Can you work these out from the model? Positions are in its coordinate system, mm. A direction names the side the tool comes from. Coordinates: 2 decimals unless noted, no trailing zeros. Write each loop counter-clockwise with the first axis right and the second up, starting at its lowest first coordinate (ties: lowest second). Pieces come first, ordered by that corner, then holes. Notation, with made-up numbers: (-7.75, 79) - (51.25, 79) arc R26 ccw to (51.25, 95) - close; hole circle Ø7 at (-1, 31). An arc over 180 degrees is marked (long way). Use one line per item in the form item = value. Start each with the question number.
(1) If I drill on probe 1 along Y at (x, z) = (0, 2); probe 2 along X at (y, z) = (-8.5, -2.5); probe 3 along X at (y, z) = (-17, 2), over which ranges is the centre line in solid material (lowest first)? Write a range as from..to.
(2) If we section it at A-A on y = -11: Please give me the cut outline in (x, z), then the cut area to 3 significant figures.
(3) If we section it at B-B on z = -2: Give the number of separate pieces and of enclosed holes in the cut face, then the cut area to 3 significant figures.
(4) Thinking about a two-plate mould opening in X: for faces 1 (the face through (14.449, 24.567, 3.586)), 2 (the face through (-3.938, -29.365, -1.972)), 3 (the face through (12.93, 21.98, 3.59)), which applies, pulls with the +X half, pulls with the -X half, needs draft (parallel to the pull), parting line crosses it, or undercut?
(5) On a 3-axis mill with a long thin cutter (end or side, diameter ignored), from which of +Z, -Z, +X, -X, +Y, -Y can I reach the whole of each face in a straight line? I mean faces 4 (the face through (12.572, -22.187, 3.586)), 5 (the face through (17.749, 20.954, 2.098)), 6 (the face through (27, 0, 3)), 7 (the face through (-27.4, -11, -2)), 8 (the face through (3.583, 28.415, -1.972)). Say none if no direction works.
(6) If we section it at D-D on y = -3.5: Please give me the cut outline in (x, z), then the cut area to 3 significant figures.
(7) If we section it at C-C on x = -3.5: Please give me the cut outline in (y, z).
(8) For pin 1 Ø0.9 at (x, y) = (27, 1) entering from -Z; pin 2 Ø2 at (y, z) = (9, -2) entering from +X; pin 3 Ø1.2 at (y, z) = (-10, -2.5) entering from -X, each with a flat end and sliding along its axis, tell me the tip position at first contact or that it passes through.
```python
from build123d import *

# Parameters (mm, degrees)
BOSS_EXTRUDE1_DEPTH = 4.34
CUT_EXTRUDE1_DEPTH  = 66.960864154
CUT_EXTRUDE2_REACH  = 73.855
CUT_EXTRUDE3_REACH  = 73.855
BOSS_EXTRUDE2_DEPTH = 4


with BuildPart() as part:
    # Sketch1 → Boss-Extrude1 (new body)
    with BuildSketch(Plane(origin=(0, 0, 0), x_dir=(0, 1, 0), z_dir=(0, 0, 1))):
        Polygon((32.908965344, 0), (16.454482672, 28.5), (-16.454482672, 28.5), (-32.908965344, 0), (-16.454482672, -28.5), (16.454482672, -28.5), align=None)
        Polygon((29.444863729, 0), (14.722431864, 25.5), (-14.722431864, 25.5), (-29.444863729, 0), (-14.722431864, -25.5), (14.722431864, -25.5), align=None, mode=Mode.SUBTRACT)
    extrude(amount=BOSS_EXTRUDE1_DEPTH)

    # Sketch2 → Cut-Extrude1 (cut, through all)
    with BuildSketch(Plane.YZ.offset(28.5)):
        with BuildLine():
            Line((-2.75, 3), (2.75, 3))
            ThreePointArc((2.75, 3), (5.75, 0), (2.75, -3))
            Line((2.75, -3), (-2.75, -3))
            ThreePointArc((-2.75, -3), (-5.75, 0), (-2.75, 3))
        make_face()
    extrude(amount=-CUT_EXTRUDE1_DEPTH, mode=Mode.SUBTRACT)

    # Cut-Extrude2: up to this face of the body (flat: up to its plane)
    cut_extrude2_end = Plane(part.part.faces().sort_by_distance((-14.25, -24.681724008, 2.17))[0])
    # Sketch3 → Cut-Extrude2 (cut, up to the picked face)
    with BuildSketch(Plane(origin=(14.25, 24.681724008, 0), x_dir=(-0.866025403784439, 0.4999999999999994, 0), z_dir=(0.4999999999999994, 0.866025403784439, 0)), mode=Mode.PRIVATE) as cut_extrude2_sk1:
        with BuildLine():
            Line((-2.75, 3), (2.75, 3))
            ThreePointArc((2.75, 3), (5.75, 0), (2.75, -3))
            Line((2.75, -3), (-2.75, -3))
            ThreePointArc((-2.75, -3), (-5.75, 0), (-2.75, 3))
        make_face()
    cut_extrude2_tool1 = split(extrude(cut_extrude2_sk1.sketch, amount=-CUT_EXTRUDE2_REACH, mode=Mode.PRIVATE), bisect_by=cut_extrude2_end, keep=Keep.BOTH, mode=Mode.PRIVATE)
    add(cut_extrude2_tool1.solids().sort_by(Axis((14.25, 24.681724, 0), (-0.4999999999999994, -0.866025403784439, 0)))[0], mode=Mode.SUBTRACT)

    # Cut-Extrude3: up to this face of the body (flat: up to its plane)
    cut_extrude3_end = Plane(part.part.faces().sort_by_distance((14.25, -24.681724008, 2.17))[0])
    # Sketch4 → Cut-Extrude3 (cut, up to the picked face)
    with BuildSketch(Plane(origin=(-14.25, 24.681724008, 0), x_dir=(-0.8660254037844384, -0.5000000000000004, 0), z_dir=(-0.5000000000000004, 0.8660254037844384, 0)), mode=Mode.PRIVATE) as cut_extrude3_sk1:
        with BuildLine():
            Line((-2.75, 3), (2.75, 3))
            ThreePointArc((2.75, 3), (5.75, 0), (2.75, -3))
            Line((2.75, -3), (-2.75, -3))
            ThreePointArc((-2.75, -3), (-5.75, 0), (-2.75, 3))
        make_face()
    cut_extrude3_tool1 = split(extrude(cut_extrude3_sk1.sketch, amount=-CUT_EXTRUDE3_REACH, mode=Mode.PRIVATE), bisect_by=cut_extrude3_end, keep=Keep.BOTH, mode=Mode.PRIVATE)
    add(cut_extrude3_tool1.solids().sort_by(Axis((-14.25, 24.681724, 0), (0.5000000000000004, -0.8660254037844384, 0)))[0], mode=Mode.SUBTRACT)

    # Sketch5 → Boss-Extrude2 (add)
    with BuildSketch(Plane(origin=(0, 0, 0), x_dir=(0, 1, 0), z_dir=(0, 0, 1))):
        Polygon((-20.304096064, 19.632274016), (-19.43807066, 19.132274016), (-15.242047107, 26.4), (-6.85, 26.4), (-6.85, 27.4), (-15.819397376, 27.4), align=None)
        Polygon((20.304096064, 19.632274016), (15.819397376, 27.4), (6.85, 27.4), (6.85, 26.4), (15.242047107, 26.4), (19.43807066, 19.132274016), align=None)
        Polygon((27.154096064, -7.767725984), (31.638794752, 0), (27.154096064, 7.767725984), (26.28807066, 7.267725984), (30.484094213, 0), (26.28807066, -7.267725984), align=None)
        Polygon((6.85, -27.4), (15.819397376, -27.4), (20.304096064, -19.632274016), (19.43807066, -19.132274016), (15.242047107, -26.4), (6.85, -26.4), align=None)
        Polygon((-20.304096064, -19.632274016), (-15.819397376, -27.4), (-6.85, -27.4), (-6.85, -26.4), (-15.242047107, -26.4), (-19.43807066, -19.132274016), align=None)
        Polygon((-27.154096064, 7.767725984), (-31.638794752, 0), (-27.154096064, -7.767725984), (-26.28807066, -7.267725984), (-30.484094213, 0), (-26.28807066, 7.267725984), align=None)
    extrude(amount=-BOSS_EXTRUDE2_DEPTH)


solid = part.part
```
Reported:
q1.probe_1 = -32.91..-29.44, 29.44..32.91
q1.probe_2 = -27.4..-26.4, 26.4..27.4
q1.probe_3 = -27.56..-21.56, 21.56..27.56
q2.outline = (-28.5, 0) - (-27.4, 0) - (-27.4, -4) - (-26.4, -4) - (-26.4, 0) - (-25.5, 0) - (-25.5, 4.34) - (-28.5, 4.34) - close; (25.5, 0) - (26.4, 0) - (26.4, -4) - (27.4, -4) - (27.4, 0) - (28.5, 0) - (28.5, 4.34) - (25.5, 4.34) - close
q2.area = 34.0 mm2
q3.separate_pieces = 6
q3.enclosed_holes = 0
q3.area = 104 mm2
q4.face_1 = pulls with the +X half
q4.face_2 = pulls with the -X half
q4.face_3 = undercut
q5.face_4 = +Z, -Z
q5.face_5 = -Z, +Y
q5.face_6 = -Z, +X, -X
q5.face_7 = -Z, -X, +Y, -Y
q5.face_8 = -Z
q6.outline = (-28.5, 2.9) - (-25.5, 2.9) - (-25.5, 4.34) - (-28.5, 4.34) - close; (25.5, 2.9) - (28.5, 2.9) - (28.5, 4.34) - (25.5, 4.34) - close
q6.area = 8.61 mm2
q7.outline = (-30.89, 0) - (-29.62, 0) - (-29.62, -4) - (-28.46, -4) - (-28.46, 0) - (-27.42, 0) - (-27.42, 4.34) - (-30.89, 4.34) - close; (27.42, 0) - (28.46, 0) - (28.46, -4) - (29.62, -4) - (29.62, 0) - (30.89, 0) - (30.89, 4.34) - (27.42, 4.34) - close
q8.pin_1 = 3
q8.pin_2 = 27.4
q8.pin_3 = -27.4
